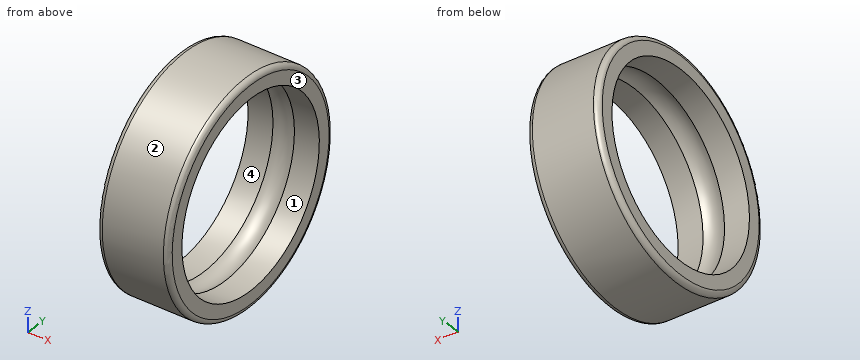
```python
from build123d import *


with BuildPart() as part:
    # Esquisse1 → Base-Révolution (revolve)
    with BuildSketch(Plane.XY, mode=Mode.PRIVATE) as base_r_volution_sk:
        with BuildLine():
            Line((1.053565375, 9.2), (3.5, 9.2))
            Line((3.5, 9.2), (3.5, 10.5))
            ThreePointArc((3.5, 10.5), (3.353553391, 10.853553391), (3, 11))
            Line((3, 11), (-3, 11))
            ThreePointArc((-3, 11), (-3.353553391, 10.853553391), (-3.5, 10.5))
            Line((-3.5, 10.5), (-3.5, 9.2))
            Line((-3.5, 9.2), (-1.053565375, 9.2))
            ThreePointArc((-1.053565375, 9.2), (0, 9.5), (1.053565375, 9.2))
        make_face()
    revolve(base_r_volution_sk.sketch.rotate(Axis((-4.370908092, 0, 0), (1, 0, 0)), 90), axis=Axis((-4.370908092, 0, 0), (1, 0, 0)))


solid = part.part
```
Geometry check sheet. Reference: the model listing, model coordinates, mm. Face numbers are marked on the shaded views. Give positions to 0.01 mm unless a question says otherwise; leave off trailing zeros. Loops run counter-clockwise (first coordinate to the right, second up) from the corner with the lowest first, then second, coordinate; pieces in that order, holes last. Notation, with made-up numbers: (78.5, 76) - (136.5, 76) arc R22 cw to (136.5, 105) - close; hole circle Ø10 at (-13, 50.5). An arc over 180 degrees is marked (long way). Use CSV: the item, a comma, the result in double quotes. Start each with the question number.
Q1. Go/stop test with flat-tipped pins: pin 1 Ø12 at (y, z) = (2, -8.5) entering from +X; pin 2 Ø2 at (x, z) = (1, -8) entering from -Y; pin 3 Ø3 at (x, y) = (2.5, 5) entering from +Z; pin 4 Ø2 at (y, z) = (-7.5, 2.5) entering from -X. Record where each tip stops, or that it passes through.
Q2. Release check for a two-part mould opening along Z. For the marked faces 1, 2, 3 and 4 record: +Z half, -Z half, draft (parallel to the pull), parting line (faces both ways), or undercut.
Q3. Scan lines: probe 1 along Y at (x, z) = (2.1, 0); probe 2 along Z at (x, y) = (-0.5, -5.5); probe 3 along Y at (x, z) = (-1.5, -1). Record each from-to range of solid material in increasing order. Write a range as from..to.
Q4. Section check D-D, the plane x = -0.25. Record the cut outline in (y, z).
Q5. Section check C-C, the plane x = 1.5. Record the cut outline in (y, z).
Q6. Section check A-A, the plane y = 0. Record the cut outline in (x, z).
Findings below:
1,pin 1,"stops at x = 3.5"
1,pin 2,"stops at y = -8.49"
1,pin 3,"stops at z = 10.43"
1,pin 4,"passes through"
2,face 1,"undercut"
2,face 2,"parting line"
2,face 3,"draft"
2,face 4,"undercut"
3,probe 1,"y = -11..-9.2, 9.2..11"
3,probe 2,"z = -9.53..-7.67, 7.67..9.53"
3,probe 3,"y = -10.95..-9.15, 9.15..10.95"
4,outline,"circle Ø22 at (0, 0); hole circle Ø18.97 at (0, 0)"
5,outline,"circle Ø22 at (0, 0); hole circle Ø18.4 at (0, 0)"
6,outline,"(-3.5, -10.5) arc R0.5 ccw to (-3, -11) - (3, -11) arc R0.5 ccw to (3.5, -10.5) - (3.5, -9.2) - (1.05, -9.2) arc R2 cw to (-1.05, -9.2) - (-3.5, -9.2) - close; (-3.5, 9.2) - (-1.05, 9.2) arc R2 cw to (1.05, 9.2) - (3.5, 9.2) - (3.5, 10.5) arc R0.5 ccw to (3, 11) - (-3, 11) arc R0.5 ccw to (-3.5, 10.5) - close"
